Part model, mm, in its own coordinate system. A direction names the side the tool comes from. Round coordinates to 2 decimals unless told otherwise and drop trailing zeros. Loops run counter-clockwise (first coordinate to the right, second up) from the corner with the lowest first, then second, coordinate; pieces in that order, holes last.
(1) Cut at B-B on z = -0.5. Count the separate pieces of the cut face and the enclosed holes in it, then the cut area to 3 significant figures.
(2) Tool access for faces 1 (the face through (86, 1.588, 0)), 2 (the face through (-2, 1, -4.762)): list every direction of +Z, -Z, +X, -X, +Y, -Y with a clear straight run to the whole face (end or side of a thin tool).
(3) Cut at A-A on x = -84. List the corners of the cut face in (y, z).
(4) Mould opens along X. For faces 3 (the face through (148.19, 3.25, 1.37)), 4 (the face through (-57, -5.398, 0)) say: +X half, -X half, draft (parallel to the pull), parting line (faces both ways), or undercut.
(5) Probe probe 1 along Z at (x, y) = (146.05, -3.5); probe 2 along Y at (x, z) = (31, -1); probe 3 along X at (y, z) = (3, -3.75) (3 decimals). List the from-to ranges inside material, lowest first.
(6) Flat gauge pins, fed straight in: pin 1 (5 mm diameter, centred on x = -87, z = 1, fed in from -Y); pin 2 (5 mm diameter, centred on x = 48.5, y = -1.5, fed in from +Z). Where does each tip first touch, or does it go through?
Autodesk Inventor part; units mm, degrees
ref_plane "Work Plane1" through (0, 5.4102, 0) normal (0, 1, 0) x (-1, 0, 0)
ref_plane "YZ Plane" through (0, 0, 0) normal (1, 0, 0) x (0, 1, 0)
ref_plane "XY Plane" through (0, 0, 0) normal (0, 0, 1) x (1, 0, 0)
sketch "Sketch1" plane through (0, 0, 0) normal (0, 0, 1) x (1, 0, 0)
  line L0 (0, 7.5565) -> (0, -7.5565)
  line L1 (-224.4725, 0) -> (224.4725, 0)
  line L2 (160.3375, -5.3975) -> (-160.3375, -5.3975)
  line L3 (-160.3375, -5.3975) -> (-160.3375, 5.3975)
  line L4 (-160.3375, 5.3975) -> (160.3375, 5.3975)
  line L5 (160.3375, 5.3975) -> (160.3375, -5.3975)
  line L6 (160.3375, -5.3975) -> (-160.3375, 5.3975) construction
  line L7 (-160.3375, -5.3975) -> (160.3375, 5.3975) construction
  point P0 (0, 0)
  dimension "d0" = 320.675
  dimension "d1" = 10.795
extrude "Extrusion1" add sketch "Sketch1" along normal mid plane 9.525
sketch "Sketch2" plane through (0, 0, 0) normal (0, 0, 1) x (1, 0, 0)
  line L0 (-160.3375, 5.3975) -> (-160.3375, -5.3975)
  line L1 (-160.3375, -5.3975) -> (160.3375, -5.3975)
  line L2 (-160.3375, -5.3975) -> (160.3375, -5.3975)
  line L3 (160.3375, -5.3975) -> (160.3375, 5.3975)
  line L4 (160.3375, 5.3975) -> (-160.3375, 5.3975)
  line L5 (-160.3375, 5.3975) -> (-160.3375, -5.3975)
  line L6 (160.3375, -5.3975) -> (160.3375, 5.3975)
  line L7 (0, 7.5565) -> (0, -7.5565)
  line L8 (-139.7, -5.3975) -> (-120.65, -5.3975)
  line L9 (-120.65, -5.3975) -> (-120.65, 1.5875)
  line L10 (-120.65, 1.5875) -> (-139.7, 1.5875)
  line L11 (-139.7, 1.5875) -> (-139.7, -5.3975)
  line L12 (-107.95, -5.3975) -> (-63.5, -5.3975)
  line L13 (-63.5, -5.3975) -> (-63.5, 1.5875)
  line L14 (-63.5, 1.5875) -> (-107.95, 1.5875)
  line L15 (-107.95, 1.5875) -> (-107.95, -5.3975)
  line L16 (160.3375, 5.3975) -> (-160.3375, 5.3975) construction
  line L17 (-112.2997, -5.3975) -> (-116.3003, -5.3975) construction
  line L18 (-116.3003, -5.3975) -> (-116.3003, 5.3975) construction
  line L19 (-116.3003, 5.3975) -> (-112.2997, 5.3975) construction
  line L20 (-112.2997, 5.3975) -> (-112.2997, -5.3975) construction
  line L21 (-112.2997, -5.3975) -> (-116.3003, 5.3975) construction
  line L22 (-116.3003, -5.3975) -> (-112.2997, 5.3975) construction
  line L23 (-144.0497, -5.3975) -> (-148.0502, -5.3975) construction
  line L24 (-148.0502, -5.3975) -> (-148.0502, 5.3975) construction
  line L25 (-148.0502, 5.3975) -> (-144.0497, 5.3975) construction
  line L26 (-144.0497, 5.3975) -> (-144.0497, -5.3975) construction
  line L27 (-144.0497, -5.3975) -> (-148.0502, 5.3975) construction
  line L28 (-148.0502, -5.3975) -> (-144.0497, 5.3975) construction
  line L29 (2.0003, -5.3975) -> (-2.0002, -5.3975) construction
  line L30 (-2.0002, -5.3975) -> (-2.0003, 5.3975) construction
  line L31 (-2.0003, 5.3975) -> (2.0002, 5.3975) construction
  line L32 (2.0002, 5.3975) -> (2.0003, -5.3975) construction
  line L33 (2.0003, -5.3975) -> (-2.0003, 5.3975) construction
  line L34 (-2.0002, -5.3975) -> (2.0002, 5.3975) construction
  line L35 (116.3003, -5.3975) -> (112.2997, -5.3975) construction
  line L36 (112.2997, -5.3975) -> (112.2997, 5.3975) construction
  line L37 (112.2997, 5.3975) -> (116.3003, 5.3975) construction
  line L38 (116.3003, 5.3975) -> (116.3003, -5.3975) construction
  line L39 (116.3003, -5.3975) -> (112.2997, 5.3975) construction
  line L40 (112.2997, -5.3975) -> (116.3003, 5.3975) construction
  line L41 (148.0503, -5.3975) -> (144.0498, -5.3975) construction
  line L42 (144.0498, -5.3975) -> (144.0498, 5.3975) construction
  line L43 (144.0498, 5.3975) -> (148.0503, 5.3975) construction
  line L44 (148.0503, 5.3975) -> (148.0503, -5.3975) construction
  line L45 (148.0503, -5.3975) -> (144.0498, 5.3975) construction
  line L46 (144.0498, -5.3975) -> (148.0503, 5.3975) construction
  line L47 (-50.8, -5.3975) -> (-6.35, -5.3975)
  line L48 (-6.35, -5.3975) -> (-6.35, 1.5875)
  line L49 (-6.35, 1.5875) -> (-50.8, 1.5875)
  line L50 (-50.8, 1.5875) -> (-50.8, -5.3975)
  point P0 (0, 0)
  point P1 (-114.3, 0)
  point P2 (-146.05, 0)
  point P3 (114.3, 0)
  point P4 (146.05, 0)
  dimension "d4" = 320.675
  dimension "d5" = 4.0005
  dimension "d6" = 114.3
  dimension "d7" = 4.0005
  dimension "d8" = 31.75
  dimension "d9" = 4.0005
  dimension "d10" = 4.0005
  dimension "d11" = 114.3
  dimension "d12" = 4.0005
  dimension "d13" = 31.75
  dimension "d14" = 6.985
  dimension "d15" = 6.35
  dimension "d16" = 6.35
  dimension "d17" = 6.35
  dimension "d19" = 6.985
  dimension "d20" = 6.35
  dimension "d21" = 19.05
  dimension "d22" = 12.7
extrude "Extrusion2" cut sketch "Sketch2" along normal up to surface (9.525 mm away) from surface at -4.7625 contours L11 L10 L9 L1 | L1 L50 L49 L48 | L15 L14 L13 L1
chamfer "Chamfer1" distance 6.35 angle 45 1 edges at (-160.3375, 5.3975, 0)
mirror "Mirror1" about plane through (0, 0, 0) normal (1, 0, 0) of "Extrusion2"
fillet "Fillet1" radius 3.175 12 edges at (-139.7, 1.5875, 0) (-120.65, 1.5875, 0) (-107.95, 1.5875, 0) (-63.5, 1.5875, 0) (-50.8, 1.5875, 0) (-6.35, 1.5875, 0) (6.35, 1.5875, 0) (50.8, 1.5875, 0) (63.5, 1.5875, 0) (107.95, 1.5875, 0) (120.65, 1.5875, 0) (139.7, 1.5875, 0)
chamfer "Chamfer2" distance 6.35 angle 45 1 edges at (160.3375, 5.3975, 0)
fillet "Fillet2" radius 3.175 4 edges at (153.9875, 5.3975, 0) (160.3375, -0.9525, 0) (-160.3375, -0.9525, 0) (-153.9875, 5.3975, 0)
ref_plane "Work Plane1" through (0, 5.4102, 0) normal (0, 1, 0) x (-1, 0, 0)
sketch "Sketch3" plane through (0, 5.4102, 0) normal (0, 1, 0) x (-1, 0, 0)
  line L0 (0, -204.47) -> (0, 204.47)
  line L1 (-204.47, 0) -> (204.47, 0)
  point P0 (0, 0)
  point P1 (114.3, 0)
  point P2 (146.05, 0)
  point P3 (0, 0)
  point P4 (-146.05, 0)
  point P5 (-114.3, 0)
  dimension "d34" = 31.75
  dimension "d35" = 114.3
  dimension "d36" = 31.75
  dimension "d37" = 114.3
hole "Hole1" at (-114.3, 5.4102, 0) at (-146.05, 5.4102, 0) at (0, 5.4102, 0) at (146.05, 5.4102, 0) at (114.3, 5.4102, 0) direction (0, -1, 0) diameter 4.8006 end through all countersink diameter 9.398 countersink angle 90
properties part number "J005229" material "ACRYLIC, CLEAR"
Final values:
1. separate pieces: 6
1. enclosed holes: 0
1. area: 1,660 mm2
2. face 1: +Z, -Z, -Y
2. face 2: -Z, +X, -X, +Y, -Y
3. outline: (1.59, -4.76) - (5.4, -4.76) - (5.4, 4.76) - (1.59, 4.76) - close
4. face 3: undercut
4. face 4: draft
5. probe 1: z = -4.76 to -2.4, 2.4 to 4.76
5. probe 2: y = 1.59 to 5.4
5. probe 3: x = -156.385 to 156.385
6. pin 1: stops at y = 1.59
6. pin 2: stops at z = 4.76
